Autodesk Inventor part; units mm, degrees
ref_plane "YZ Plane" through (0, 0, 0) normal (1, 0, 0) x (0, 1, 0)
ref_plane "XZ Plane" through (0, 0, 0) normal (0, 1, 0) x (-1, 0, 0)
ref_plane "XY Plane" through (0, 0, 0) normal (0, 0, 1) x (1, 0, 0)
sketch "Esquisse1" plane through (0, 0, 0) normal (0, 0, 1) x (1, 0, 0)
  line L0 (-8.5, -10) -> (-3.5, -10)
  line L1 (-3.5, -10) -> (-3.5, -9.5)
  line L2 (-3.5, -9.5) -> (-3, -9.5)
  line L3 (-3, -9.5) -> (-3, -8.3)
  line L4 (-3, -8.3) -> (-5.2994, -8.3)
  arc A0 (-5.7944, -7.105) -> (-5.2994, -8.3) centre (-5.2994, -7.6) ccw
  line L5 (-5.7944, -7.105) -> (-2.1755, -3.4861)
  arc A1 (-1.6076, -3.388) -> (-2.1755, -3.4861) centre (-1.8219, -3.8397) ccw
  arc A2 (-1.6076, -3.388) -> (-0.3, -3.738) centre (0, 0) ccw
  line L6 (-0.3, -3.738) -> (0, -3.45)
  line L7 (0, -3.45) -> (0.3, -3.738)
  arc A3 (0.3, -3.738) -> (1.6076, -3.388) centre (0, 0) ccw
  arc A4 (2.1755, -3.4861) -> (1.6076, -3.388) centre (1.8219, -3.8397) ccw
  line L8 (2.1755, -3.4861) -> (5.7944, -7.105)
  arc A5 (5.2994, -8.3) -> (5.7944, -7.105) centre (5.2994, -7.6) ccw
  line L9 (5.2994, -8.3) -> (3, -8.3)
  line L10 (3, -8.3) -> (3, -9.5)
  line L11 (3, -9.5) -> (3.5, -9.5)
  line L12 (3.5, -9.5) -> (3.5, -10)
  line L13 (3.5, -10) -> (8.5, -10)
  arc A6 (8.5, -10) -> (10, -8.5) centre (8.5, -8.5) ccw
  line L14 (10, -8.5) -> (10, -3.5)
  line L15 (10, -3.5) -> (9.5, -3.5)
  line L16 (9.5, -3.5) -> (9.5, -3)
  line L17 (9.5, -3) -> (8.3, -3)
  line L18 (8.3, -3) -> (8.3, -5.2994)
  arc A7 (7.105, -5.7944) -> (8.3, -5.2994) centre (7.6, -5.2994) ccw
  line L19 (7.105, -5.7944) -> (3.4861, -2.1755)
  arc A8 (3.388, -1.6076) -> (3.4861, -2.1755) centre (3.8397, -1.8219) ccw
  arc A9 (3.388, -1.6076) -> (3.738, -0.3) centre (0, 0) ccw
  line L20 (3.738, -0.3) -> (3.45, 0)
  line L21 (3.45, 0) -> (3.738, 0.3)
  arc A10 (3.738, 0.3) -> (3.388, 1.6076) centre (0, 0) ccw
  arc A11 (3.4861, 2.1755) -> (3.388, 1.6076) centre (3.8397, 1.8219) ccw
  line L22 (3.4861, 2.1755) -> (7.105, 5.7944)
  arc A12 (8.3, 5.2994) -> (7.105, 5.7944) centre (7.6, 5.2994) ccw
  line L23 (8.3, 5.2994) -> (8.3, 3)
  line L24 (8.3, 3) -> (9.5, 3)
  line L25 (9.5, 3) -> (9.5, 3.5)
  line L26 (9.5, 3.5) -> (10, 3.5)
  line L27 (10, 3.5) -> (10, 8.5)
  arc A13 (10, 8.5) -> (8.5, 10) centre (8.5, 8.5) ccw
  line L28 (8.5, 10) -> (3.5, 10)
  line L29 (3.5, 10) -> (3.5, 9.5)
  line L30 (3.5, 9.5) -> (3, 9.5)
  line L31 (3, 9.5) -> (3, 8.3)
  line L32 (3, 8.3) -> (5.2994, 8.3)
  arc A14 (5.7944, 7.105) -> (5.2994, 8.3) centre (5.2994, 7.6) ccw
  line L33 (5.7944, 7.105) -> (2.1755, 3.4861)
  arc A15 (1.6076, 3.388) -> (2.1755, 3.4861) centre (1.8219, 3.8397) ccw
  arc A16 (1.6076, 3.388) -> (0.3, 3.738) centre (0, 0) ccw
  line L34 (0.3, 3.738) -> (0, 3.45)
  line L35 (0, 3.45) -> (-0.3, 3.738)
  arc A17 (-0.3, 3.738) -> (-1.6076, 3.388) centre (0, 0) ccw
  arc A18 (-2.1755, 3.4861) -> (-1.6076, 3.388) centre (-1.8219, 3.8397) ccw
  line L36 (-2.1755, 3.4861) -> (-5.7944, 7.105)
  arc A19 (-5.2994, 8.3) -> (-5.7944, 7.105) centre (-5.2994, 7.6) ccw
  line L37 (-5.2994, 8.3) -> (-3, 8.3)
  line L38 (-3, 8.3) -> (-3, 9.5)
  line L39 (-3, 9.5) -> (-3.5, 9.5)
  line L40 (-3.5, 9.5) -> (-3.5, 10)
  line L41 (-3.5, 10) -> (-8.5, 10)
  arc A20 (-8.5, 10) -> (-10, 8.5) centre (-8.5, 8.5) ccw
  line L42 (-10, 8.5) -> (-10, 3.5)
  line L43 (-10, 3.5) -> (-9.5, 3.5)
  line L44 (-9.5, 3.5) -> (-9.5, 3)
  line L45 (-9.5, 3) -> (-8.3, 3)
  line L46 (-8.3, 3) -> (-8.3, 5.2994)
  arc A21 (-7.105, 5.7944) -> (-8.3, 5.2994) centre (-7.6, 5.2994) ccw
  line L47 (-7.105, 5.7944) -> (-3.4861, 2.1755)
  arc A22 (-3.388, 1.6076) -> (-3.4861, 2.1755) centre (-3.8397, 1.8219) ccw
  arc A23 (-3.388, 1.6076) -> (-3.738, 0.3) centre (0, 0) ccw
  line L48 (-3.738, 0.3) -> (-3.45, 0)
  line L49 (-3.45, 0) -> (-3.738, -0.3)
  arc A24 (-3.738, -0.3) -> (-3.388, -1.6076) centre (0, 0) ccw
  arc A25 (-3.4861, -2.1755) -> (-3.388, -1.6076) centre (-3.8397, -1.8219) ccw
  line L50 (-3.4861, -2.1755) -> (-7.105, -5.7944)
  arc A26 (-8.3, -5.2994) -> (-7.105, -5.7944) centre (-7.6, -5.2994) ccw
  line L51 (-8.3, -5.2994) -> (-8.3, -3)
  line L52 (-8.3, -3) -> (-9.5, -3)
  line L53 (-9.5, -3) -> (-9.5, -3.5)
  line L54 (-9.5, -3.5) -> (-10, -3.5)
  line L55 (-10, -3.5) -> (-10, -8.5)
  arc A27 (-10, -8.5) -> (-8.5, -10) centre (-8.5, -8.5) ccw
  circle A28 centre (0, 0) radius 2.4
  dimension "d2" = 4.8
extrude "Extrusion1" add sketch "Esquisse1" along normal mid plane 268.3
properties part number "Profilés du réduit 20x20"
The model under review builds one solid part; all positions refer to its coordinate system, in mm. Give positions to 0.01 mm unless a question says otherwise; leave off trailing zeros. Put each result on its own line as item: value.
(1) For pin 1 Ø0.6 at (y, z) = (-10, 49) entering from +X; pin 2 Ø0.6 at (x, z) = (10, -64.5) entering from -Y; pin 3 Ø0.6 at (y, z) = (9, -63.5) entering from +X, all flat-tipped, find the tip position at first contact; note any pin that passes through.
Results are:
pin 1: x = 9.4
pin 2: y = -9.4
pin 3: x = 9.99
(2) The part is to be moulded in two halves that separate along X. For faces 1 (the cylindrical face through (1.29, -2.024, -1.878)), 2 (the flat face through (-10, 6, -2)), 3 (the flat face through (10, -6, -2)), say which applies: pulls with the +X half, pulls with the -X half, needs draft (parallel to the pull), parting line crosses it, or undercut.
Results are:
face 1: undercut
face 2: pulls with the -X half
face 3: pulls with the +X half
(3) To check wall thickness, follow probe 1 along X at (y, z) = (0.5, 53.5); probe 2 along Y at (x, z) = (0, 1.5); probe 3 along Y at (x, z) = (-5.5, 67). State the ranges of each line that lie inside material, in increasing order. Write a range as from..to.
Results are:
probe 1: -3.72..-2.35, 2.35..3.72
probe 2: -3.45..-2.4, 2.4..3.45
probe 3: -10..-8.27, -6.81..-4.19, 4.19..6.81, 8.27..10
